```python
from build123d import *

# Parameters (mm, degrees)
F0_W              = 1219.2
F0_H              = 609.6
F1_DEPTH          = 1.51892
F2_W              = 1219.2
F2_H              = 609.6
F2_W_2            = 1216.16216
F2_H_2            = 606.56216
F3_DEPTH          = 38.1
F5_DEPTH          = 685.8
F7_W              = 1219.2
F7_H              = 609.6
F8_DEPTH          = 1.51892
F9_W              = 1219.2
F9_H              = 609.6
F9_W_2            = 1213.12432
F9_H_2            = 603.52432
F10_DEPTH         = 38.1
F11_W             = 101.6
F11_H             = 609.6
F12_DEPTH         = 1.51892
F13_R             = 1.5875
F14_DEPTH         = 1.651
F14_COPIES2_COUNT = 2
F14_COPIES2_PITCH = 1240.259203
F16_D             = 6.35


# Not quite as in the source:
# - a pattern or mirror of a feature is missing from the dataset's text; its kind, count and spacing are read off the source's solid


with BuildPart() as f1:
    # F0 (on Top) → F1 (new body)
    with BuildSketch(Plane.XY):
        Rectangle(F0_W, F0_H)
    extrude(amount=-F1_DEPTH)

    # F2 (on face) → F3 (join)
    with BuildSketch(Plane(origin=(0, 0, -1.51892), x_dir=(1, 0, 0), z_dir=(0, 0, -1))):
        Rectangle(F2_W, F2_H)
        Rectangle(F2_W_2, F2_H_2, mode=Mode.SUBTRACT)
    extrude(amount=F3_DEPTH)

    # F4 (on face) → F5 (join)
    with BuildSketch(Plane(origin=(0, 0, -1.51892), x_dir=(1, 0, 0), z_dir=(0, 0, -1))):
        Polygon((-571.5, 301.76216), (-571.5, 304.8), (-609.6, 304.8), (-609.6, 266.7), (-606.56216, 266.7), (-606.56216, 301.76216), align=None)
        Polygon((571.5, 304.8), (571.5, 301.76216), (606.56216, 301.76216), (606.56216, 266.7), (609.6, 266.7), (609.6, 304.8), align=None)
    f5 = extrude(amount=F5_DEPTH)

    # F5_copies: F5 across plane
    add(f5.mirror(Plane.ZX))

    # F7 (on offset) → F8 (join)
    with BuildSketch(Plane.XY.offset(-647.7)):
        Rectangle(F7_W, F7_H)
    extrude(amount=-F8_DEPTH)

    # F9 (on face) → F10 (join)
    with BuildSketch(Plane(origin=(0, 0, -649.21892), x_dir=(1, 0, 0), z_dir=(0, 0, -1))):
        Rectangle(F9_W, F9_H)
        Rectangle(F9_W_2, F9_H_2, mode=Mode.SUBTRACT)
    extrude(amount=F10_DEPTH)

    # F11 (on face) → F12 (join)
    with BuildSketch(Plane(origin=(0, 0, -687.31892), x_dir=(1, 0, 0), z_dir=(0, 0, -1))):
        with Locations((-558.8, 0)):
            Rectangle(F11_W, F11_H)
    f12 = extrude(amount=F12_DEPTH)

    # F12_copies: F12 across plane
    add(f12.mirror(Plane(origin=(0, 0, 0), x_dir=(0, 0, 1), z_dir=(1, 0, 0))))

    # F13 (on face) → F14 (cut)
    with BuildSketch(Plane(origin=(0, 0, -688.83784), x_dir=(1, 0, 0), z_dir=(0, 0, -1))):
        with Locations((-596.9, 292.1)):
            Circle(F13_R)
        with Locations((-596.9, 225.425)):
            Circle(F13_R)
        with Locations((-530.225, 292.1)):
            Circle(F13_R)
        with Locations((-530.225, 225.425)):
            Circle(F13_R)
    f14 = extrude(amount=-F14_DEPTH, mode=Mode.SUBTRACT)

    # F14_copies: F14 across plane
    add(f14.mirror(Plane(origin=(0, 0, 0), x_dir=(0, 0, 1), z_dir=(1, 0, 0))), mode=Mode.SUBTRACT)

    # F14_copies1: F14 across plane
    add(f14.mirror(Plane.ZX), mode=Mode.SUBTRACT)

    # F14_copies2: F14 ×2
    with Locations(*[Vector(0.9087818071, 0.4172716466, 0) * (i * F14_COPIES2_PITCH) for i in range(1, F14_COPIES2_COUNT)]):
        add(f14, mode=Mode.SUBTRACT)

    # F16 (through all)
    with Locations(Plane.XZ.offset(304.8)):
        with Locations((-501.65, -19.812), (-463.55, -19.812)):
            Hole(F16_D / 2)


solid = f1.part
```
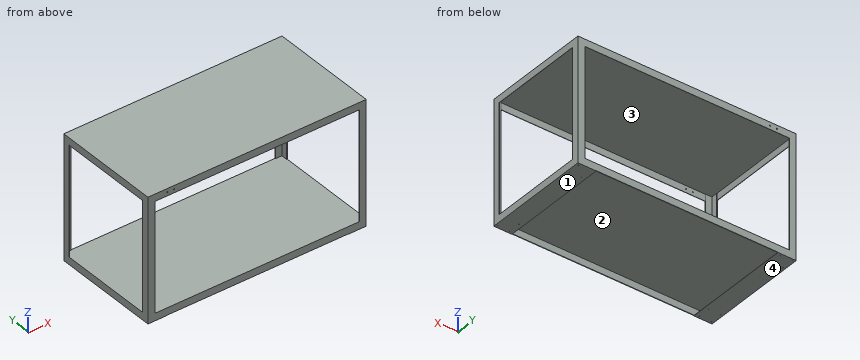
Model file for the job. Use its own axes, mm. Face numbers are marked on the shaded views. A direction names the side the tool comes from. Round coordinates to 2 decimals unless told otherwise and drop trailing zeros. Write each loop counter-clockwise with the first axis right and the second up, starting at its lowest first coordinate (ties: lowest second). Pieces come first, ordered by that corner, then holes. Notation, with made-up numbers: (11.25, -3) - (23.25, -3) arc R14 cw to (23.25, 14) - close; hole circle Ø4 at (-34, -6). An arc over 180 degrees is marked (long way). One line per item, written item: value.
(1) Two-plate mould, pull along Y, no slides. Class the marked faces 3 and 4: pulls with the +Y half, pulls with the -Y half, needs draft (parallel to the pull), parting line crosses it, or undercut.
Values follow:
face 3: undercut
face 4: needs draft
(2) 3-axis set-ups, long thin cutter, end or side, ignore diameter. For the marked faces 1 and 2: which of +Z, -Z, +X, -X, +Y, -Y reach the whole face in a straight line?
Values follow:
face 1: -Z, +X, -X, +Y, -Y
face 2: none
(3) Drop flat-ended pins along their axis: P1, Ø12, axis at x = -368, y = -133.5, coming from the -Z side; P2, Ø3.5, axis at x = -147, y = -303.5, coming from the -Z side. Give the stop position or say it passes through.
Values follow:
P1: stops at z = -649.22
P2: stops at z = -687.32
(4) Cut at C-C, the plane x = -58.5. Give the cut face in (y, z), plus the area to 3 significant figures.
Values follow:
outline: (-304.8, -687.32) - (-301.76, -687.32) - (-301.76, -649.22) - (301.76, -649.22) - (301.76, -687.32) - (304.8, -687.32) - (304.8, -647.7) - (-304.8, -647.7) - close; (-304.8, -39.62) - (-303.28, -39.62) - (-303.28, -1.52) - (303.28, -1.52) - (303.28, -39.62) - (304.8, -39.62) - (304.8, 0) - (-304.8, 0) - close
area: 2,200 mm²
(5) Wall check: probe 1 along Y at (x, z) = (-596.9, -688.2); probe 2 along X at (y, z) = (-292, -688); probe 3 along Z at (x, y) = (-517, 46). Give the ranges that are in metal, low to high.
Values follow:
probe 1: y = -304.8 to -293.69, -290.51 to -227.01, -223.84 to 223.84, 227.01 to 290.51, 293.69 to 304.8
probe 2: x = -609.6 to -598.48, -595.32 to -531.81, -528.64 to -508, 508 to 528.64, 531.81 to 595.32, 598.48 to 609.6
probe 3: z = -688.84 to -687.32, -649.22 to -647.7, -1.52 to 0
(6) Cut at A-A, the plane z = -253.5. Give the cut face in (x, y).
Values follow:
outline: (-609.6, -304.8) - (-571.5, -304.8) - (-571.5, -301.76) - (-606.56, -301.76) - (-606.56, -266.7) - (-609.6, -266.7) - close; (-609.6, 266.7) - (-606.56, 266.7) - (-606.56, 301.76) - (-571.5, 301.76) - (-571.5, 304.8) - (-609.6, 304.8) - close; (571.5, -304.8) - (609.6, -304.8) - (609.6, -266.7) - (606.56, -266.7) - (606.56, -301.76) - (571.5, -301.76) - close; (571.5, 301.76) - (606.56, 301.76) - (606.56, 266.7) - (609.6, 266.7) - (609.6, 304.8) - (571.5, 304.8) - close
(7) Cut at B-B, the plane y = -2.5. Give the cut face in (x, z), plus the area to 3 significant figures.
Values follow:
outline: (-609.6, -688.84) - (-508, -688.84) - (-508, -687.32) - (-606.56, -687.32) - (-606.56, -649.22) - (606.56, -649.22) - (606.56, -687.32) - (508, -687.32) - (508, -688.84) - (609.6, -688.84) - (609.6, -647.7) - (-609.6, -647.7) - close; (-609.6, -39.62) - (-608.08, -39.62) - (-608.08, -1.52) - (608.08, -1.52) - (608.08, -39.62) - (609.6, -39.62) - (609.6, 0) - (-609.6, 0) - close
area: 4,360 mm²
